Autodesk Fusion 360 part; units mm, degrees
sketch "Schizzo1" plane through (0, 0, 0) normal (0, 0, 1) x (1, 0, 0)
  line L0 (4.5367, 58.7959) -> (119.2367, 58.7959) construction
  line L1 (119.2367, 58.7959) -> (119.2367, 5.0959) construction
  line L2 (119.2367, 5.0959) -> (4.5367, 5.0959) construction
  line L3 (4.5367, 5.0959) -> (4.5367, 58.7959) construction
  line L4 (4.5367, 31.9459) -> (119.2367, 31.9459) construction
  line L5 (61.8867, 58.7959) -> (61.8867, 5.0959) construction
  line L6 (119.1367, 5.1959) -> (4.6367, 5.1959)
  line L7 (4.6367, 5.1959) -> (4.6367, 58.6959)
  line L8 (4.6367, 58.6959) -> (119.1367, 58.6959)
  line L9 (119.1367, 58.6959) -> (119.1367, 5.1959)
  line L10 (117.2367, 7.0959) -> (6.5367, 7.0959)
  line L11 (6.5367, 7.0959) -> (6.5367, 56.7959)
  line L12 (6.5367, 56.7959) -> (117.2367, 56.7959)
  line L13 (117.2367, 56.7959) -> (117.2367, 7.0959)
  line L14 (6.5367, 56.7959) -> (34.5367, 56.7959)
  line L15 (34.5367, 56.7959) -> (34.5367, 46.7959)
  line L16 (34.5367, 46.7959) -> (6.5367, 46.7959)
  line L17 (6.5367, 46.7959) -> (6.5367, 56.7959)
  line L18 (73.5367, 56.7959) -> (73.5367, 46.7959)
  line L19 (73.5367, 46.7959) -> (45.5367, 46.7959)
  line L20 (45.5367, 46.7959) -> (45.5367, 56.7959)
  line L21 (45.5367, 56.7959) -> (73.5367, 56.7959)
  line L22 (4.5367, 36.9459) -> (119.1367, 36.9459)
  line L23 (4.5367, 26.9459) -> (119.1367, 26.9459)
  line L24 (61.8867, 58.7959) -> (61.8867, 5.0959)
  line L25 (112.5367, 56.7959) -> (112.5367, 46.7959)
  line L26 (112.5367, 46.7959) -> (84.5367, 46.7959)
  line L27 (84.5367, 46.7959) -> (84.5367, 56.7959)
  line L28 (84.5367, 56.7959) -> (112.5367, 56.7959)
  line L29 (37.5367, 58.7959) -> (37.5367, 5.0959)
  line L30 (42.5367, 58.7959) -> (42.5367, 5.0959)
  line L31 (76.5367, 58.7959) -> (76.5367, 5.0959)
  line L32 (81.5367, 58.6959) -> (81.5367, 5.0959)
  dimension "d1" = 114.7
  dimension "d2" = 53.7
  dimension "d3" = 0.1
  dimension "d6" = 2
  dimension "d7" = 28
  dimension "d8" = 10
  dimension "d11" = 39
  dimension "d12" = 0
  dimension "d15" = 10
  dimension "d38" = 5
  dimension "d39" = 3
  dimension "d40" = 5
  dimension "d41" = 3
extrude "Estrusione1" add sketch "Schizzo1" along normal blind 1 contours L10 L13 L23 L32 | L10 L23 L31 L32 | L13 L22 L23 L32 | L10 L23 L24 L31 | L22 L23 L31 L32 | L12 L13 L22 L25 L26 L27 L32 | L10 L23 L24 L30 | L22 L23 L24 L31 | L12 L22 L31 L32 | L10 L23 L29 L30 | L22 L23 L24 L30 | L12 L18 L19 L22 L24 L31 | L10 L11 L23 L29 | L22 L23 L29 L30 | L12 L19 L20 L22 L24 L30 | L11 L22 L23 L29 | L12 L22 L29 L30 | L11 L12 L15 L16 L22 L29
extrude "Estrusione2" add sketch "Schizzo1" along normal blind 4 contours L6 L9 L10 L13 L23 L32 | L6 L10 L31 L32 | L9 L13 L22 L23 | L6 L10 L24 L31 | L8 L9 L12 L13 L22 L28 L32 | L13 L22 L23 L32 | L6 L10 L24 L30 | L22 L23 L31 L32 | L6 L10 L29 L30 | L22 L23 L24 L31 | L8 L12 L31 L32 | L6 L7 L10 L11 L23 L29 | L22 L23 L24 L30 | L8 L12 L21 L24 L31 | L22 L23 L29 L30 | L8 L12 L21 L24 L30 | L7 L11 L22 L23 | L11 L22 L23 L29 | L8 L12 L29 L30 | L7 L8 L11 L12 L14 L17 L22 L29
fillet "Raccordo1" radius 3 4 edges at (4.6367, 5.1959, 2) (119.1367, 5.1959, 2) (119.1367, 58.6959, 2) (4.6367, 58.6959, 2)
ref_plane "Piano di lavoro1" through (61.8867, 31.9459, 0) normal (-1, 0, 0) x (0, -1, 0)
sketch "Schizzo3" plane through (61.8867, 0, 0) normal (-1, 0, 0) x (0, -1, 0)
  line L0 (-26.9459, 4) -> (-36.9459, 4) construction
  line L1 (-36.9459, 4) -> (-36.9459, 0) construction
  line L2 (-36.9459, 0) -> (-26.9459, 0) construction
  line L3 (-26.9459, 0) -> (-26.9459, 4) construction
  line L4 (-55.6959, 4) -> (-8.1959, 4) construction
  line L5 (-58.7959, 0) -> (-5.0959, 0) construction
  line L6 (-26.9459, 1) -> (-26.9459, 4) construction
  line L7 (-36.9459, 1) -> (-36.9459, 4) construction
  line L8 (-31.9459, 4) -> (-31.9459, 0) construction
  line L9 (-26.9459, 1) -> (-36.9459, 1) construction
  line L10 (-26.9459, 1) -> (-26.9459, 4)
  line L11 (-26.9459, 4) -> (-28.678, 1)
  line L12 (-28.678, 1) -> (-26.9459, 1)
  line L13 (-36.9459, 1) -> (-36.9459, 4)
  line L14 (-36.9459, 4) -> (-35.2139, 1)
  line L15 (-35.2139, 1) -> (-36.9459, 1)
  dimension "d20" = 30
extrude "Estrusione4" cut sketch "Schizzo3" along normal mid plane 110
sketch "Schizzo4" plane through (0, 0, 4) normal (0, 0, 1) x (-1, 0, 0)
  arc A0 (-7.6367, -58.6959) -> (-4.6367, -55.6959) centre (-7.6367, -55.6959) ccw
  line L0 (-4.6367, -55.6959) -> (-4.6367, -8.1959)
  arc A1 (-4.6367, -8.1959) -> (-7.6367, -5.1959) centre (-7.6367, -8.1959) ccw
  line L1 (-7.6367, -5.1959) -> (-116.1367, -5.1959)
  arc A2 (-116.1367, -5.1959) -> (-119.1367, -8.1959) centre (-116.1367, -8.1959) ccw
  line L2 (-119.1367, -8.1959) -> (-119.1367, -55.6959)
  arc A3 (-119.1367, -55.6959) -> (-116.1367, -58.6959) centre (-116.1367, -55.6959) ccw
  line L3 (-116.1367, -58.6959) -> (-7.6367, -58.6959)
  line L4 (-117.2367, -36.9459) -> (-116.8867, -36.9459)
  line L5 (-116.8867, -36.9459) -> (-6.8867, -36.9459)
  line L6 (-6.8867, -36.9459) -> (-6.5367, -36.9459)
  line L7 (-6.5367, -36.9459) -> (-6.5367, -56.7959)
  line L8 (-6.5367, -56.7959) -> (-117.2367, -56.7959)
  line L9 (-117.2367, -56.7959) -> (-117.2367, -36.9459)
  line L10 (-117.2367, -7.0959) -> (-6.5367, -7.0959)
  line L11 (-6.5367, -7.0959) -> (-6.5367, -26.9459)
  line L12 (-6.5367, -26.9459) -> (-6.8867, -26.9459)
  line L13 (-6.8867, -26.9459) -> (-116.8867, -26.9459)
  line L14 (-117.2367, -26.9459) -> (-117.2367, -7.0959)
  line L15 (-4.6367, -58.6959) -> (-119.1367, -58.6959) construction
  line L16 (-119.1367, -58.6959) -> (-119.1367, -5.1959) construction
  line L17 (-119.1367, -5.1959) -> (-4.6367, -5.1959) construction
  line L18 (-4.6367, -5.1959) -> (-4.6367, -58.6959) construction
  line L19 (-49.2367, -58.6959) -> (-58.2367, -58.6959)
  line L20 (-58.2367, -58.6959) -> (-58.2367, -5.1959)
  line L21 (-58.2367, -5.1959) -> (-49.2367, -5.1959)
  line L22 (-49.2367, -5.1959) -> (-49.2367, -58.6959)
  line L23 (-65.2367, -58.6959) -> (-74.2367, -58.6959)
  line L24 (-74.2367, -58.6959) -> (-74.2367, -5.1959)
  line L25 (-74.2367, -5.1959) -> (-65.2367, -5.1959)
  line L26 (-65.2367, -5.1959) -> (-65.2367, -58.6959)
  line L27 (-53.7367, -58.6959) -> (-53.7367, -5.1959) construction
  line L28 (-69.7367, -58.6959) -> (-69.7367, -5.1959) construction
  line L29 (-2.7367, -58.6959) -> (-2.7367, -5.1959) construction
  line L30 (-116.8867, -26.9459) -> (-117.2367, -26.9459)
  dimension "d28" = 9
  dimension "d29" = 9
  dimension "d33" = 1.9
  dimension "d34" = 51
  dimension "d35" = 67
extrude "Estrusione6" cut sketch "Schizzo4" against normal blind 2 contours L3 L8 L19 L20 L22 | L5 L8 L20 L22 | L3 L8 L23 L24 L26 | L5 L13 L20 L22 | L1 L10 L20 L21 L22 | L5 L8 L24 L26 | L10 L13 L20 L22 | L5 L13 L24 L26 | L1 L10 L24 L25 L26 | L10 L13 L24 L26
extrude "Estrusione7" add sketch "Schizzo1" along normal blind 4 contours L10 L23 L31 L32 | L22 L23 L31 L32 | L12 L22 L31 L32 | L10 L23 L29 L30 | L22 L23 L29 L30 | L12 L22 L29 L30
Source: CAD feature listing. Evaluate the final solid. Frame: model axes, mm. A direction names the side the tool comes from. Give positions to 0.01 mm unless a question says otherwise; leave off trailing zeros. Order: outer loops, then holes, each group sorted by start corner. A loop starts at its lowest first (then second) coordinate and runs counter-clockwise, first axis right, second up. Notation, with made-up numbers: (46.5, 77) -> (56.5, 77) arc R17 cw to (56.5, 105) -> close; hole circle Ø3 at (67.25, 73.25). An arc over 180 degrees is marked (long way). Write item = value, one per line.
Q1. Pin query (flat end, axial travel): pin 1 (11 mm diameter, centred on x = 53, y = 18, fed in from +Z); pin 2 (1 mm diameter, centred on x = 54.5, y = 6.5, fed in from +Z); pin 3 (2 mm diameter, centred on y = 58, z = 3.5, fed in from +X). Return the tip coordinate at first contact, or that it passes through.
Data:
pin_1 = 1
pin_2 = 2
pin_3 = 118.84
Q2. Set-up query: faces 1 (the face through (100, 7.096, 2)), 2 (the face through (49.237, 6, 3)), 3 (the face through (59.77, 35.9, 2.19)). Return all of +Z, -Z, +X, -X, +Y, -Y with unobstructed straight access to the full face (end or side cutting, diameter ignored); none if empty.
Data:
face_1 = +Z
face_2 = +Z, +Y, -Y
face_3 = none
Q3. Cut plane D-D, the plane y = 24.5. Output: boundary loops of the cut face in (x, z).
Data:
outline = (4.64, 0) -> (119.14, 0) -> (119.14, 4) -> (117.24, 4) -> (117.24, 1) -> (81.54, 1) -> (81.54, 4) -> (76.54, 4) -> (76.54, 1) -> (42.54, 1) -> (42.54, 4) -> (37.54, 4) -> (37.54, 1) -> (6.54, 1) -> (6.54, 4) -> (4.64, 4) -> close
Q4. Material intervals for line 1 (X direction, y = 29, z = 3.6); line 2 (X direction, y = 53, z = 0.25); line 3 (X direction, y = 46.5, z = 3.55), sorted ascending. Write a range as from..to.
Data:
line_1 = 4.64..49.24, 58.24..65.24, 74.24..119.14
line_2 = 4.64..6.54, 34.54..45.54, 73.54..84.54, 112.54..119.14
line_3 = 4.64..6.54, 37.54..42.54, 76.54..81.54, 117.24..119.14
Q5. Cut plane A-A, the plane x = 99. Output: boundary loops of the cut face in (y, z), and give its area (3 significant figures).
Data:
outline = (5.2, 0) -> (46.8, 0) -> (46.8, 1) -> (35.21, 1) -> (36.95, 4) -> (26.95, 4) -> (28.68, 1) -> (7.1, 1) -> (7.1, 4) -> (5.2, 4) -> close; (56.8, 0) -> (58.7, 0) -> (58.7, 4) -> (56.8, 4) -> close
area = 79.7 mm^2
Q6. Cut plane C-C, the plane z = 3.15. State how many separate pieces and enclosed holes the cut face has, and give its area (3 significant figures).
Data:
separate_pieces = 5
enclosed_holes = 4
area = 1,790 mm^2
Q7. Cut plane B-B, the plane y = 30. Output: boundary loops of the cut face in (x, z).
Data:
outline = (4.64, 0) -> (119.14, 0) -> (119.14, 4) -> (74.24, 4) -> (74.24, 2) -> (65.24, 2) -> (65.24, 4) -> (58.24, 4) -> (58.24, 2) -> (49.24, 2) -> (49.24, 4) -> (4.64, 4) -> close
Q8. Pull-direction query (X, two-part tool) for faces 4 (the face through (42.537, 18, 2)), 5 (the face through (28, 32, 4)), 6 (the face through (5.49, 6.1, 2.03)); classes: released by +X, released by -X, zero draft, split by the parting line, or undercut.
Data:
face_4 = undercut
face_5 = zero draft
face_6 = released by -X
